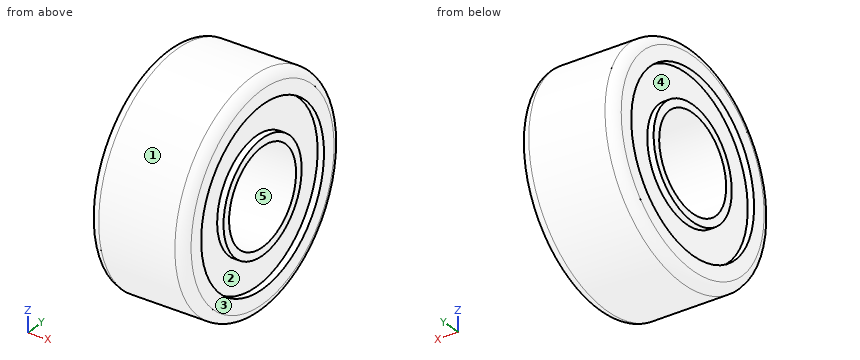
Autodesk Inventor part; units mm, degrees
ref_plane "YZ Plane" through (0, 0, 0) normal (1, 0, 0) x (0, 1, 0)
ref_plane "XZ Plane" through (0, 0, 0) normal (0, 1, 0) x (-1, 0, 0)
ref_plane "XY Plane" through (0, 0, 0) normal (0, 0, 1) x (1, 0, 0)
sketch "スケッチ1" plane through (0, 0, 0) normal (1, 0, 0) x (0, 1, 0)
  circle A0 centre (0, 0) radius 3.5
  dimension "d0" = 7
extrude "押し出し1" add sketch "スケッチ1" along normal blind 3
sketch "スケッチ2" plane through (3, 0, 0) normal (1, 0, 0) x (0, 0, -1)
  circle A0 centre (0, 0) radius 1.5
  dimension "d3" = 3
extrude "押し出し2" cut sketch "スケッチ2" against normal blind 3
sketch "スケッチ3" plane through (3, 0, 0) normal (1, 0, 0) x (0, 0, -1)
  circle A0 centre (0, 0) radius 1.75
  circle A1 centre (0, 0) radius 2.75
  dimension "d6" = 3.5
  dimension "d7" = 5.5
extrude "押し出し3" cut sketch "スケッチ3" against normal blind 0.2
sketch "スケッチ4" plane through (0, 0, 0) normal (-1, 0, 0) x (0, 0, 1)
  circle A0 centre (0, 0) radius 1.75
  circle A1 centre (0, 0) radius 2.75
  dimension "d10" = 3.5
  dimension "d11" = 5.5
extrude "押し出し4" cut sketch "スケッチ4" against normal blind 0.2
fillet "フィレット1" radius 0.3 1 edges at (3, -3.5, 0)
fillet "フィレット2" radius 0.3 1 edges at (0, -3.5, 0)
properties part number "d7_bearing" material "鋼、合金"
Design review of the part built by this model. Coordinates are the model's own, in mm. Face numbers are marked on the shaded views. A direction names the side the tool comes from. Coordinates: 2 decimals unless noted, no trailing zeros. Order: outer loops, then holes, each group sorted by start corner. A loop starts at its lowest first (then second) coordinate and runs counter-clockwise, first axis right, second up. Notation, with made-up numbers: M 26.25,15 L 54.25,15 A23 ccw 54.25,42 Z; hole C 67.25,-1 d2. An arc over 180 degrees is marked long. Answer as a JSON object with one key per item and string values. Group by question number.
1) Add section C-C, the plane x = 1.25. Write out the cut boundary in (y, z), then the cut area to 3 significant figures.
2) Add section A-A, the plane z = 0. Write out the cut boundary in (x, y).
3) For pin 1 (1.6 mm diameter, centred on y = -0.5, z = 0, fed in from +X), flat-tipped, find the tip position at first contact; note if it passes through.
4) Wall thickness on L1, parallel to Y at x = 0.9, z = 1; L2, parallel to X at y = -2.25, z = -0.75: over which ranges is each line inside the solid? List them lowest first.
5) Mouldability with a two-part tool opening along Y and no side actions: class the marked faces 1, 2 and 3 as pulls with the +Y half, pulls with the -Y half, needs draft (parallel to the pull), parting line crosses it, or undercut.
6) Tool access review of the marked faces 4 and 5: name each direction out of +Z, -Z, +X, -X, +Y, -Y from which nothing blocks a thin tool from reaching the whole face with its end or side.
Computed values:
{
 "1": {"outline": "C 0,0 d7; hole C 0,0 d3", "area": "31.4 mm^2"},
 "2": {"outline": "M 0,-3.2 A0.3 ccw 0.3,-3.5 L 2.7,-3.5 A0.3 ccw 3,-3.2 L 3,-2.75 L 2.8,-2.75 L 2.8,-1.75 L 3,-1.75 L 3,-1.5 L 0,-1.5 L 0,-1.75 L 0.2,-1.75 L 0.2,-2.75 L 0,-2.75 Z; M 0,1.5 L 3,1.5 L 3,1.75 L 2.8,1.75 L 2.8,2.75 L 3,2.75 L 3,3.2 A0.3 ccw 2.7,3.5 L 0.3,3.5 A0.3 ccw 0,3.2 L 0,2.75 L 0.2,2.75 L 0.2,1.75 L 0,1.75 Z"},
 "3": {"pin 1": "passes through"},
 "4": {"L1": "y = -3.35 to -1.12, 1.12 to 3.35", "L2": "x = 0.2 to 2.8"},
 "5": {"face 1": "parting line crosses it", "face 2": "undercut", "face 3": "needs draft"},
 "6": {"face 4": "-X", "face 5": "+X, -X"}
}
